from build123d import *

# Parameters (mm, degrees)
F0_W     = 38.1
F0_H     = 12.7
F0_W_2   = 12.7
F0_H_2   = 3.175
F1_DEPTH = 3.175
F2_DEPTH = 15.24
F3_R     = 6.34999
F4_R     = 3.81
F5_R     = 1.5875
F6_DEPTH = 12.701
F7_R     = 2.54
F8_DEPTH = 3.176


# Not quite as in the source:
# - a fillet or chamfer is up to 0.001 mm smaller than in the source, because OpenCascade refuses the exact size


with BuildPart() as f1:
    # F0 (on Top) → F1 (new body)
    with BuildSketch(Plane.XY):
        Rectangle(F0_W, F0_H)
        Rectangle(F0_W_2, F0_H_2, mode=Mode.SUBTRACT)
    extrude(amount=F1_DEPTH)

    # F0 (on Top) → F2 (join)
    with BuildSketch(Plane.XY):
        Rectangle(F0_W_2, F0_H_2)
    extrude(amount=F2_DEPTH)

    # F3 (radius 6.35 in the source; OpenCascade refuses exactly that, so slightly less here)
    f3_edges = [f1.edges().sort_by_distance(p)[0] for p in [
        (-6.35, 0, 15.24),
        (6.35, 0, 15.24),
    ]]
    fillet(f3_edges, radius=F3_R)

    # F4 (call 1 of 5: OpenCascade refuses the feature's edges together)
    f4_edges = [f1.edges().sort_by_distance(p)[0] for p in [
        (-19.05, -6.35, 1.5875),
    ]]
    fillet(f4_edges, radius=F4_R)

    # F4#2 (call 2 of 5)
    f4_2_edges = [f1.edges().sort_by_distance(p)[0] for p in [
        (-19.05, 6.35, 1.5875),
    ]]
    fillet(f4_2_edges, radius=F4_R)

    # F4#3 (call 3 of 5)
    f4_3_edges = [f1.edges().sort_by_distance(p)[0] for p in [
        (19.05, 6.35, 1.5875),
    ]]
    fillet(f4_3_edges, radius=F4_R)

    # F4#4 (call 4 of 5)
    f4_4_edges = [f1.edges().sort_by_distance(p)[0] for p in [
        (19.05, -6.35, 1.5875),
    ]]
    fillet(f4_4_edges, radius=F4_R)

    # F4#5 (call 5 of 5)
    f4_5_edges = [f1.edges().sort_by_distance(p)[0] for p in [
        (0, -1.5875, 3.175),
        (0, 1.5875, 3.175),
        (6.35, 0, 3.175),
        (-6.35, 0, 3.175),
    ]]
    fillet(f4_5_edges, radius=F4_R)

    # F5 (on face) → F6 (cut, through all)
    with BuildSketch(Plane.XZ.offset(6.35)):
        with Locations((0, 11.2299183384)):
            Circle(F5_R)
    extrude(amount=-F6_DEPTH, mode=Mode.SUBTRACT)

    # F7 (on face) → F8 (cut, through all)
    with BuildSketch(Plane.XY.offset(3.175)):
        with Locations((-13.97, 0)):
            Circle(F7_R)
        with Locations((13.97, 0)):
            Circle(F7_R)
    extrude(amount=-F8_DEPTH, mode=Mode.SUBTRACT)


solid = f1.part
Read the model definition and answer for the solid it produces. Units are mm, in the model's axes. A direction names the side the tool comes from. Give positions to 0.01 mm unless a question says otherwise; leave off trailing zeros. Write each loop counter-clockwise with the first axis right and the second up, starting at its lowest first coordinate (ties: lowest second). Pieces come first, ordered by that corner, then holes. Notation, with made-up numbers: (69.25, 28) -> (76.25, 28) arc R17 ccw to (76.25, 58) -> close; hole circle Ø3 at (22, 32.5). An arc over 180 degrees is marked (long way). Answer as a JSON object with one key per item and string values. Group by question number.
1) Find section A-A (x = -13.97). Write down the section's boundary in (y, z) (3 decimals).
2) Each of these flat-tipped pins is pushed along its axis until it touches: P1, Ø5, axis at x = 2.5, z = 5, coming from the -Y side; P2, Ø4, axis at x = 13.97, y = 0, coming from the -Z side; P3, Ø6, axis at x = -13.97, y = 0, coming from the +Z side (3 decimals); P4, Ø4, axis at x = 0, z = 13, coming from the -Y side. Where does it stop, or does it pass through?
3) Find section C-C (z = 10.75). Write down the section's boundary in (x, y).
4) The mould has two halves that part along X. Classify faces 1 (the cylindrical face through (-0.207, -0.022, 12.804)), 2 (the cylindrical face through (-16.508, 0.112, 1.61)), 3 (the flat face through (0, -6.35, 2)), 4 (the cylindrical face through (8.01, 0.08, 3.84)): +X half, -X half, draft (parallel to the pull), parting line (faces both ways), or undercut.
5) Find section B-B (y = 0). Count the separate pieces of the cut face and the enclosed holes in it, and give its area (3 significant figures).
6) A tool of negligible diameter and unlimited length cuts with its end or side. For faces 5 (the flat face through (-6.35, 0, 8)), 6 (the flat face through (0, -6, 3.175)), 7 (the flat face through (0, 0, 0)), from which of +Z, -Z, +X, -X, +Y, -Y can it reach the whole face along a straight path? Write none if from no direction.
7) Consider L1, parallel to Z at x = 0, y = -0.1; L2, parallel to X at y = 1.5, z = 2.5; L3, parallel to Y at x = -13.97, z = 0.7. Determine where each line is inside the solid, lowest interval first. Write a range as from..to.
Values follow:
{
 "1": {"outline": "(-6.35, 0) -> (-2.54, 0) -> (-2.54, 3.175) -> (-6.35, 3.175) -> close; (2.54, 0) -> (6.35, 0) -> (6.35, 3.175) -> (2.54, 3.175) -> close"},
 "2": {"P1": "stops at y = -6.35", "P2": "passes through", "P3": "stops at z = 3.175", "P4": "stops at y = -1.59"},
 "3": {"outline": "(-6.07, -1.59) -> (-1.51, -1.59) -> (-1.51, 1.59) -> (-6.07, 1.59) -> close; (1.51, -1.59) -> (6.07, -1.59) -> (6.07, 1.59) -> (1.51, 1.59) -> close"},
 "4": {"face 1": "undercut", "face 2": "undercut", "face 3": "draft", "face 4": "+X half"},
 "5": {"separate pieces": "3", "enclosed holes": "1", "area": "223 mm2"},
 "6": {"face 5": "+Z, -X, +Y, -Y", "face 6": "+Z", "face 7": "-Z, +X, -X, +Y, -Y"},
 "7": {"L1": "z = 0..9.64, 12.82..15.24", "L2": "x = -19.05..-16.02, -11.92..11.92, 16.02..19.05", "L3": "y = -6.35..-2.54, 2.54..6.35"}
}
